from build123d import *

# Parameters (mm, degrees)
SKETCH1_RX          = 244
SKETCH1_RY          = 110
BOSS_EXTRUDE1_DEPTH = 3
SKETCH12_R          = 6.83635542
CUT_EXTRUDE8_DEPTH  = 4
SKETCH13_W          = 488
SKETCH13_H          = 5
SKETCH13_H_2        = 15
CUT_EXTRUDE9_DEPTH  = 4
CUT_EXTRUDE10_DEPTH = 10
CUT_EXTRUDE11_DEPTH = 10
CHAMFER1_SIZE       = 10


with BuildPart() as part:
    # Sketch1 → Boss-Extrude1 (new body)
    with BuildSketch(Plane.XY):
        with Locations((0, 0)):
            Ellipse(SKETCH1_RX, SKETCH1_RY)
    extrude(amount=-BOSS_EXTRUDE1_DEPTH)

    # Sketch12 → Cut-Extrude8 (cut, through all)
    with BuildSketch(Plane.XY):
        with Locations((200, -30)):
            Circle(SKETCH12_R)
        with Locations((-200, -30)):
            Circle(SKETCH12_R)
    extrude(amount=-CUT_EXTRUDE8_DEPTH, mode=Mode.SUBTRACT)

    # Sketch13 → Cut-Extrude9 (cut, through all)
    with BuildSketch(Plane.XY):
        with Locations((0, -107.5)):
            Rectangle(SKETCH13_W, SKETCH13_H)
        with Locations((0, 102.5)):
            Rectangle(SKETCH13_W, SKETCH13_H_2)
    extrude(amount=-CUT_EXTRUDE9_DEPTH, mode=Mode.SUBTRACT)

    # Sketch14 → Cut-Extrude10 (cut)
    with BuildSketch(Plane.XY):
        Polygon((-76.2, -81.5), (-76.2, -93.9), (76.2, -93.9), (76.2, -81.5), (81.2, -81.5), (81.2, -78.5), (76.2, -78.5), (76.2, -15), (-76.2, -15), (-76.2, -78.5), (-81.2, -78.5), (-81.2, -81.5), align=None)
    extrude(amount=-CUT_EXTRUDE10_DEPTH, mode=Mode.SUBTRACT)

    # Sketch15 → Cut-Extrude11 (cut)
    with BuildSketch(Plane.XY):
        Polygon((-137.5, 83.1), (137.5, 83.1), (137.5, 28.1), (142.5, 28.1), (142.5, 25.1), (137.5, 25.1), (137.5, 15.1), (-137.5, 15.1), (-137.5, 25.1), (-142.5, 25.1), (-142.5, 28.1), (-137.5, 28.1), align=None)
    extrude(amount=-CUT_EXTRUDE11_DEPTH, mode=Mode.SUBTRACT)

    # Chamfer1
    chamfer1_edges = [part.edges().sort_by_distance(p)[0] for p in [
        (-137.5, 83.1, -1.5),
        (137.5, 83.1, -1.5),
    ]]
    chamfer(chamfer1_edges, length=CHAMFER1_SIZE)


solid = part.part
Design review of the part built by this model. Coordinates are the model's own, in mm. A direction names the side the tool comes from. Round coordinates to 2 decimals unless told otherwise and drop trailing zeros. Order: outer loops, then holes, each group sorted by start corner. A loop starts at its lowest first (then second) coordinate and runs counter-clockwise, first axis right, second up. Notation, with made-up numbers: M -9,28.5 L 33,28.5 A18 ccw 33,47.5 Z; hole C -19.75,35 d7. An arc over 180 degrees is marked long. Answer as CSV lines item,"result". Start each with the question number.
1) The part is to be moulded in two halves that separate along X. For faces 1 (the face through (-193.685, -32.618, -1.479)), 2 (the face through (-3, -4, -3)), say which applies: +X half, -X half, draft (parallel to the pull), parting line (faces both ways), or undercut.
2) Wall thickness on line 1 along Y through (x, z) = (-45, -1.85); line 2 along Y through (x, z) = (77, -2.75); line 3 along X through (y, z) = (32.5, -2.6): over which ranges is each line inside the solid? List them lowest first. Write a range as [from, to].
3) For pin 1 Ø0.9 at (y, z) = (59.5, -1.5) entering from +X; pin 2 Ø0.9 at (x, z) = (-79, -1.5) entering from -Y; pin 3 Ø18 at (x, y) = (200, -30) entering from -Z; pin 4 Ø1.5 at (y, z) = (21, -2) entering from -X, all flat-tipped, find the tip position at first contact; note any pin that passes through.
4) Tool access review of faces 3 (the face through (132.4, 78.2, -1.5)), 4 (the face through (-3, -4, 0)): name each direction out of +Z, -Z, +X, -X, +Y, -Y from which nothing blocks a thin tool from reaching the whole face with its end or side.
5) Add section B-B (z = -1.4). Give the number of separate pieces and of enclosed holes in the cut face, then the cut area to 3 significant figures.
6) Add section A-A (x = 16). Give the boundary of the cut face in (y, z).
Resolved:
1,face 1,"undercut"
1,face 2,"draft"
2,line 1,"[-105, -93.9], [-15, 15.1], [83.1, 95]"
2,line 2,"[-104.38, -81.5], [-78.5, 15.1], [83.1, 95]"
2,line 3,"[-233.11, -137.5], [137.5, 233.11]"
3,pin 1,"x = 205.86"
3,pin 2,"y = -104.14"
3,pin 3,"z = -3"
3,pin 4,"x = -239.83"
4,face 3,"+Z, -Z"
4,face 4,"+Z, +X, -X, +Y, -Y"
5,separate pieces,"1"
5,enclosed holes,"4"
5,area,"50,400 mm^2"
6,outline,"M -105,-3 L -93.9,-3 L -93.9,0 L -105,0 Z; M -15,-3 L 15.1,-3 L 15.1,0 L -15,0 Z; M 83.1,-3 L 95,-3 L 95,0 L 83.1,0 Z"
